```python
from build123d import *

# Parameters (mm, degrees)
SKETCH1_R           = 12.7
BOSS_EXTRUDE1_DEPTH = 25.4
SKETCH1_4_W         = 16.51
SKETCH1_4_H         = 16.51
BOSS_EXTRUDE2_DEPTH = 25.4
BOSS_EXTRUDE3_DEPTH = 12.7


with BuildPart() as part:
    # Sketch1 → Boss-Extrude1 (new body)
    with BuildSketch(Plane.XY):
        with BuildLine():
            Line((150.843809628, 46.203312203), (87.343809628, 46.203312203))
            Line((87.343809628, 46.203312203), (87.343809628, -29.996687797))
            Line((87.343809628, -29.996687797), (150.843809628, -29.996687797))
            Line((150.843809628, -29.996687797), (163.543809628, -17.296687797))
            Line((163.543809628, -17.296687797), (163.543809628, 33.503312203))
            ThreePointArc((163.543809628, 33.503312203), (159.824065749, 42.483568324), (150.843809628, 46.203312203))
        make_face()
        with Locations((138.143809628, 20.803312203)):
            Circle(SKETCH1_R, mode=Mode.SUBTRACT)
    extrude(amount=BOSS_EXTRUDE1_DEPTH)



with BuildPart() as body_2:
    # Sketch1<4> → Boss-Extrude2 (new body)
    with BuildSketch(Plane.XY):
        with Locations((44.798809628, 37.948312203)):
            Rectangle(SKETCH1_4_W, SKETCH1_4_H)
    extrude(amount=BOSS_EXTRUDE2_DEPTH)


with BuildPart() as part_1:
    add(part.part)

    add(body_2.part)  # Boss-Extrude3 merges body 2
    # Sketch1<5> → Boss-Extrude3 (add)
    with BuildSketch(Plane.XY):
        with BuildLine():
            Line((87.343809628, 46.203312203), (53.053809628, 46.203312203))
            Line((53.053809628, 46.203312203), (53.053809628, 29.693312203))
            Line((53.053809628, 29.693312203), (36.543809628, 29.693312203))
            Line((36.543809628, 29.693312203), (36.543809628, -17.296687797))
            ThreePointArc((36.543809628, -17.296687797), (40.263553507, -26.276943918), (49.243809628, -29.996687797))
            Line((49.243809628, -29.996687797), (87.343809628, -29.996687797))
            Line((87.343809628, -29.996687797), (87.343809628, 46.203312203))
        make_face()
    extrude(amount=BOSS_EXTRUDE3_DEPTH)


solid = part_1.part
```
Geometry: final body of the model. Coordinates: model frame, mm. A direction names the side the tool comes from. Round coordinates to 2 decimals unless told otherwise and drop trailing zeros. Write each loop counter-clockwise with the first axis right and the second up, starting at its lowest first coordinate (ties: lowest second). Pieces come first, ordered by that corner, then holes.
Item 1: Section query A-A (z = 23.5). Return loops of the section in (x, y).
Item 2: Section query B-B (y = -9.5). Return loops of the section in (x, z).
Item 3: Section query C-C (z = 2). Return loops of the section in (x, y).
Item 4: Set-up query: faces 1 (the face through (45, 29.693, 19)), 2 (the face through (159.922, 42.384, 12.522)), 3 (the face through (53.054, 38, 19)). Return all of +Z, -Z, +X, -X, +Y, -Y with unobstructed straight access to the full face (end or side cutting, diameter ignored); none if empty.
Item 5: Material intervals for L1, parallel to X at y = -0.5, z = 17; L2, parallel to Y at x = 149, z = 17; L3, parallel to Y at x = 136, z = 6, sorted ascending.
Item 6: Section query D-D (y = 24). Return loops of the section in (x, z).
Item 7: Pin query (flat end, axial travel): P1, Ø6.5, axis at y = 13, z = 16.5, coming from the -X side; P2, Ø14, axis at x = 46.5, z = 19.5, coming from the -Y side; P3, Ø2, axis at x = 69, y = -5, coming from the +Z side; P4, Ø1, axis at x = 90.5, y = 13, coming from the -Z side. Return the tip coordinate at first contact, or that it passes through.
Item 8: Mould query, pull axis X, two halves, no side actions, for faces 4 (the face through (62, 9, 12.7)), 5 (the face through (40.17, -26.18, 6.26)), 6 (the face through (125.456, 21.362, 12.522)), 7 (the face through (157.1, -23.74, 12.52)). Classes: +X half, -X half, draft (parallel to the pull), parting line (faces both ways), or undercut.
Completed:
1. outline: (36.54, 29.69) - (53.05, 29.69) - (53.05, 46.2) - (36.54, 46.2) - close; (87.34, -30) - (150.84, -30) - (163.54, -17.3) - (163.54, 33.5) arc R12.7 ccw to (150.84, 46.2) - (87.34, 46.2) - close; hole circle Ø25.4 at (138.14, 20.8)
2. outline: (36.54, 0) - (163.54, 0) - (163.54, 25.4) - (87.34, 25.4) - (87.34, 12.7) - (36.54, 12.7) - close
3. outline: (36.54, -17.3) arc R12.7 ccw to (49.24, -30) - (150.84, -30) - (163.54, -17.3) - (163.54, 33.5) arc R12.7 ccw to (150.84, 46.2) - (36.54, 46.2) - close; hole circle Ø25.4 at (138.14, 20.8)
4. face 1: +Z, -X, -Y
4. face 2: +Z, -Z, +X, +Y
4. face 3: +Z, +Y, -Y
5. L1: x = 87.34 to 163.54
5. L2: y = -30 to 14.21, 27.39 to 46.2
5. L3: y = -30 to 8.29, 33.32 to 46.2
6. outline: (36.54, 0) - (125.85, 0) - (125.85, 25.4) - (87.34, 25.4) - (87.34, 12.7) - (36.54, 12.7) - close; (150.43, 0) - (163.54, 0) - (163.54, 25.4) - (150.43, 25.4) - close
7. P1: stops at x = 87.34
7. P2: stops at y = -29.95
7. P3: stops at z = 12.7
7. P4: stops at z = 0
8. face 4: undercut
8. face 5: -X half
8. face 6: undercut
8. face 7: +X half
